The listing builds one solid part. Answer for the finished solid, in the listing's coordinates (mm). A direction names the side the tool comes from. Coordinates: 2 decimals unless noted, no trailing zeros. Order: outer loops, then holes, each group sorted by start corner. A loop starts at its lowest first (then second) coordinate and runs counter-clockwise, first axis right, second up. Notation, with made-up numbers: (89.5, 33.5) -> (134.5, 33.5) arc R33 cw to (134.5, 71.5) -> close; hole circle Ø7 at (88.5, -1.75). An arc over 180 degrees is marked (long way). Write item = value, one per line.
from build123d import *

# Parameters (mm, degrees)
BOSS_EXTRUDE1_DEPTH = 3.175
FILLET1_R           = 2.54


with BuildPart() as part:
    # Sketch1 → Boss-Extrude1 (new, symmetric)
    with BuildSketch(Plane.XY):
        Polygon((-8.240014, 97.536), (-8.240014, 84.582), (-5.700014, 84.582), (-5.700014, 88.011), (0, 88.011), (0, -88.011), (-5.700014, -88.011), (-5.700014, -84.582), (-8.240014, -84.582), (-8.240014, -97.536), (12.7, -97.536), (12.7, 97.536), align=None)
    extrude(amount=BOSS_EXTRUDE1_DEPTH, both=True)

    # Fillet1
    fillet1_edges = [part.edges().sort_by_distance(p)[0] for p in [
        (12.7, -97.536, 0),
        (-8.240014, -97.536, 0),
        (-8.240014, -84.582, 0),
        (12.7, 97.536, 0),
        (-8.240014, 84.582, 0),
        (-8.240014, 97.536, 0),
    ]]
    fillet(fillet1_edges, radius=FILLET1_R - 0.0001)  # a hair under: the kernel refuses the full size


solid = part.part
Q1. The mould has two halves that part along X. Classify faces 3 (the face through (2, 97.536, 0)), 4 (the face through (12.7, -1, 0)), 5 (the face through (-3, -88.011, 0)): released by +X, released by -X, zero draft, split by the parting line, or undercut.
The answers:
face_3 = zero draft
face_4 = released by +X
face_5 = undercut
Q2. Find the intervals of material crossed by line 1 along Y through (x, z) = (-1.75, 3); line 2 along Y through (x, z) = (10.25, -2); line 3 along X through (y, z) = (79, 3), in increasing order.
The answers:
line_1 = -97.54 to -88.01, 88.01 to 97.54
line_2 = -97.53 to 97.53
line_3 = 0 to 12.7
Q3. A tool of negligible diameter and unlimited length cuts with its end or side. For faces 1 (the face through (7, 1, -3.175)), 2 (the face through (-5.7, -86, 0)), from which of +Z, -Z, +X, -X, +Y, -Y can it reach the whole face along a straight path? Write none if from no direction.
The answers:
face_1 = -Z, +X, -X, +Y, -Y
face_2 = +Z, -Z
Q4. This flat-tipped pin is pushed along its axis until it touches: pin 1 Ø3 at (y, z) = (-8.5, 0.5) entering from -X. Where does it stop, or does it pass through?
The answers:
pin_1 = 0
Q5. Section B-B, the plane y = -36.5 is taken. Give the vertices of the cut face in (x, z) (3 decimals).
The answers:
outline = (0, -3.175) -> (12.7, -3.175) -> (12.7, 3.175) -> (0, 3.175) -> close
